Can you work these out from the model? Positions are in its coordinate system, mm. Face numbers are marked on the shaded views. A direction names the side the tool comes from. Coordinates: 2 decimals unless noted, no trailing zeros. Loops run counter-clockwise (first coordinate to the right, second up) from the corner with the lowest first, then second, coordinate; pieces in that order, holes last. Notation, with made-up numbers: (-3.5, 88.5) -> (32.5, 88.5) arc R17 ccw to (32.5, 100.5) -> close; hole circle Ø3 at (36.5, -24.75). An arc over 180 degrees is marked (long way). Use one line per item in the form item = value. Start each with the question number.
(1) On a 3-axis mill with a long thin cutter (end or side, diameter ignored), from which of +Z, -Z, +X, -X, +Y, -Y can I reach the whole of each face in a straight line? I mean the marked faces 4 and 5. Say none if no direction works.
(2) I'm going to push flat-ended pins straight in: pin 1 (6 mm diameter, centred on x = -54.5, y = -26.5, fed in from +Z); pin 2 (24 mm diameter, centred on x = -17.5, z = 38, fed in from -Y). Where does each tip first touch, or does it pass through?
(3) Imagine slicing it at D-D (x = 25.5). List the corners of the cut face in (y, z) for me, plus the area to 3 significant figures.
(4) Imagine slicing it at C-C (z = 42.5). State how many separate pieces and enclosed holes the cut face has, plus the area to 3 significant figures.
(5) I need wall thicknesses on line 1 (Y direction, x = 44, z = 55.5); line 2 (X direction, y = -20, z = 49.5); line 3 (Y direction, x = 56, z = 31). Which ranges of each line are inside material? Lowest first, please. Write a range as [from, to].
(6) Imagine slicing it at B-B (x = -1.5). List the corners of the cut face in (y, z) for me, plus the area to 3 significant figures.
(7) Thinking about a two-plate mould opening in X: for the marked faces 1, 2 and 3, which applies, released by +X, released by -X, zero draft, split by the parting line, or undercut?
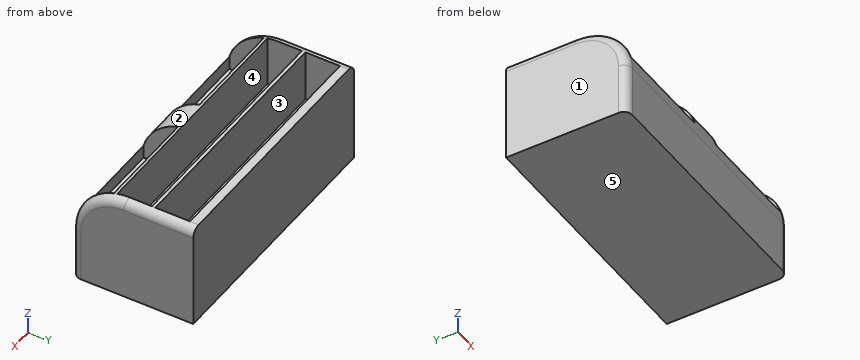
```python
from build123d import *

# Parameters (mm, degrees)
F0_W        = 150
F0_H        = 70
F0_W_2      = 60
F0_H_2      = 20
F0_W_3      = 140
F1_DEPTH    = 60
F2_T1_DEPTH = 300
F3_R        = 4.99999
F4_W        = 140
F4_H        = 20.1229466498
F4_H_2      = 20
F5_DEPTH    = 30


# Not quite as in the source:
# - a fillet or chamfer that OpenCascade refuses, or shapes differently, is made with other operations: its cross-section is extruded or revolved along the edge and cut away or added
# - a fillet or chamfer is up to 0.001 mm smaller than in the source, because OpenCascade refuses the exact size


with BuildPart() as f1:
    # F0 (on Top) → F1 (new body)
    with BuildSketch(Plane.XY):
        Rectangle(F0_W, F0_H)
        with Locations((-40, -24)):
            Rectangle(F0_W_2, F0_H_2, mode=Mode.SUBTRACT)
        with Locations((40, -24)):
            Rectangle(F0_W_2, F0_H_2, mode=Mode.SUBTRACT)
        with Locations((0, -2)):
            Rectangle(F0_W_3, F0_H_2, mode=Mode.SUBTRACT)
        with Locations((0, 20)):
            Rectangle(F0_W_3, F0_H_2, mode=Mode.SUBTRACT)
    extrude(amount=F1_DEPTH)

    # F2: fillet of radius 30 on 1 edges, made by hand

    # F2_s2 → F2_t1 (cut)
    with BuildSketch(Plane.YZ.offset(-150)):
        with BuildLine():
            ThreePointArc((-35, 30), (-26.2132034356, 51.2132034356), (-5, 60))
            Line((-5, 60), (-35, 60))
            Line((-35, 60), (-35, 30))
        make_face()
    extrude(amount=F2_T1_DEPTH, mode=Mode.SUBTRACT)

    # F3 (radius 5 in the source; OpenCascade refuses exactly that, so slightly less here)
    f3_edges = [f1.edges().sort_by_distance(p)[0] for p in [
        (75, 15, 60),
        (-75, 15, 60),
    ]]
    fillet(f3_edges, radius=F3_R)

    # F4 (on face) → F5 (join)
    with BuildSketch(Plane(origin=(0, 0, 0), x_dir=(1, 0, 0), z_dir=(0, 0, -1))):
        with Locations((0, -19.9385266751)):
            Rectangle(F4_W, F4_H)
        with Locations((0, 2)):
            Rectangle(F4_W, F4_H_2)
        with Locations((0, 24)):
            Rectangle(F4_W, F4_H_2)
    extrude(amount=-F5_DEPTH)


solid = f1.part
```
Worked out:
q1.face_4 = +Z
q1.face_5 = -Z, +X, -X, +Y, -Y
q2.pin_1 = 30
q2.pin_2 = -35
q3.outline = (-35, 0) -> (35, 0) -> (35, 60) -> (30, 60) -> (30, 30) -> (10, 30) -> (10, 60) -> (8, 60) -> (8, 30) -> (-12, 30) -> (-12, 59.17) arc R30 ccw to (-14, 58.62) -> (-14, 30) -> (-34, 30) -> (-34, 37.68) arc R30 ccw to (-35, 30) -> close
q3.area = 2,370 mm2
q4.separate_pieces = 1
q4.enclosed_holes = 2
q4.area = 2,290 mm2
q5.line_1 = [-14, -12], [8, 10], [30, 35]
q5.line_2 = [-75, -70], [-10, 10], [70, 75]
q5.line_3 = [-34.98, -34], [-14, -12], [8, 10], [30, 35]
q6.outline = (-35, 0) -> (35, 0) -> (35, 60) -> (30, 60) -> (30, 30) -> (10, 30) -> (10, 60) -> (8, 60) -> (8, 30) -> (-12, 30) -> (-12, 59.17) arc R30 ccw to (-35, 30) -> close
q6.area = 2,810 mm2
q7.face_1 = released by -X
q7.face_2 = zero draft
q7.face_3 = undercut
